from build123d import *

# Parameters (mm, degrees)
F0_R     = 40
F1_DEPTH = 5
F3_D     = 5.5
F4_SIZE  = 1


with BuildPart() as f1:
    # F0 (on Top) → F1 (new body)
    with BuildSketch(Plane.XY):
        Circle(F0_R)
    extrude(amount=F1_DEPTH)

    # F3 (through all)
    with Locations(Plane(origin=(0, 0, 0), x_dir=(1, 0, 0), z_dir=(0, 0, -1))):
        with Locations((0, 30), (25.980762, -15), (-25.980762, -15), (0, -30), (25.980762, 15), (-25.980762, 15)):
            Hole(F3_D / 2)

    # F4
    f4_edges = [f1.edges().sort_by_distance(p)[0] for p in [
        (-40, 0, 5),
        (-40, 0, 0),
    ]]
    chamfer(f4_edges, length=F4_SIZE)


solid = f1.part
Work out the finished part from the listing and answer in its coordinate system (mm). Coordinates: 2 decimals unless noted, no trailing zeros. Write each loop counter-clockwise with the first axis right and the second up, starting at its lowest first coordinate (ties: lowest second). Pieces come first, ordered by that corner, then holes. Notation, with made-up numbers: M 23,62.5 L 39,62.5 A5 cw 39,66.5 Z; hole C 61.25,-35.5 d9. An arc over 180 degrees is marked long. Use one line per item in the form item = value. Start each with the question number.
1. The part is cut by section C-C (y = -14). Give the number of separate pieces and of enclosed holes in the cut face, plus the area to 3 significant figures.
2. The part is cut by section B-B (z = 2.15). Give the vertices of the cut face in (x, y).
3. The part is cut by section A-A (x = 0). Give the vertices of the cut face in (y, z).
4. The mould has two halves that part along X. Classify faces 1 (the face through (-28.604, -15.826, 2.535)), 2 (the face through (-8.67, -39.05, 2.48)), 3 (the face through (-1, 1, 5)): released by +X, released by -X, zero draft, split by the parting line, or undercut.
5. Straight lines are drawn through the part: probe 1 along Y at (x, z) = (0, 3.15); probe 2 along Y at (x, z) = (-25, 2); probe 3 along X at (y, z) = (14, 4.75). For each, find the intervals that lie inside material, in ascending order. Write a range as from..to.
6. Each of these flat-tipped pins is pushed along its axis until it touches: P1, Ø3, axis at x = 27, y = -4, coming from the -Z side; P2, Ø3, axis at y = -6, z = 1, coming from the +X side; P3, Ø2, axis at y = -2, z = 4.5, coming from the +X side. Where does it stop, or does it pass through?
Evaluation:
q1.separate_pieces = 3
q1.enclosed_holes = 0
q1.area = 321 mm^2
q2.outline = C 0,0 d80; hole C -25.98,-15 d5.5; hole C -25.98,15 d5.5; hole C 0,-30 d5.5; hole C 0,30 d5.5; hole C 25.98,-15 d5.5; hole C 25.98,15 d5.5
q3.outline = M -40,1 L -39,0 L -32.75,0 L -32.75,5 L -39,5 L -40,4 Z; M -27.25,0 L 27.25,0 L 27.25,5 L -27.25,5 Z; M 32.75,0 L 39,0 L 40,1 L 40,4 L 39,5 L 32.75,5 Z
q4.face_1 = undercut
q4.face_2 = split by the parting line
q4.face_3 = zero draft
q5.probe_1 = -40..-32.75, -27.25..27.25, 32.75..40
q5.probe_2 = -31.22..-17.57, -12.43..12.43, 17.57..31.22
q5.probe_3 = -36.67..-28.54, -23.42..23.42, 28.54..36.67
q6.P1 = 0
q6.P2 = 39.75
q6.P3 = 39.98
